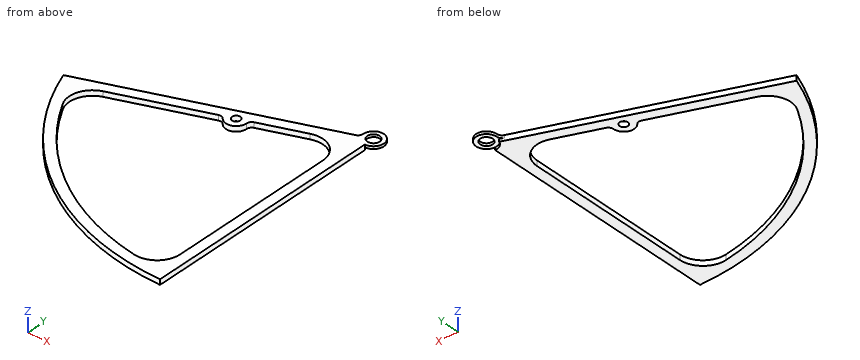
```python
from build123d import *

# Parameters (mm, degrees)
SZKIC1_R                    = 12
SZKIC1_R_2                  = 8
DODANIE_WYCI_GNI_CIE1_DEPTH = 10
SZKIC2_R                    = 20
WYTNIJ_WYCI_GNI_CIE1_DEPTH  = 5
ZAOKR_GLENIE1_R             = 45
ZAOKR_GLENIE2_R             = 10


with BuildPart() as part:
    # Szkic1 → Dodanie-wyciągnięcie1 (new body)
    with BuildSketch(Plane.XY):
        with BuildLine():
            Line((0, -20), (0, -490))
            ThreePointArc((0, -490), (-281.052453812, -401.384501702), (-460.449384185, -167.58987023))
            Line((-460.449384185, -167.58987023), (-18.793852416, -6.840402867))
            ThreePointArc((-18.793852416, -6.840402867), (11.471528727, 16.383040886), (0, -20))
        make_face()
        Circle(SZKIC1_R, mode=Mode.SUBTRACT)
        with Locations((-190.094997116, -90.472476083)):
            Circle(SZKIC1_R_2, mode=Mode.SUBTRACT)
        with BuildLine():
            Line((-20, -28.562960135), (-20, -469.574275275))
            ThreePointArc((-20, -469.574275275), (-269.580925085, -385.001460816), (-434.41507852, -179.397713347))
            Line((-434.41507852, -179.397713347), (-208.888849532, -97.312878949))
            ThreePointArc((-208.888849532, -97.312878949), (-183.254594249, -109.266328498), (-171.3011447, -83.632073216))
            Line((-171.3011447, -83.632073216), (-20, -28.562960135))
        make_face(mode=Mode.SUBTRACT)
    extrude(amount=DODANIE_WYCI_GNI_CIE1_DEPTH)

    # Szkic2 → Wytnij-wyciągnięcie1 (cut)
    with BuildSketch(Plane(origin=(0, 0, 0), x_dir=(-1, 0, 0), z_dir=(0, 0, -1))):
        Circle(SZKIC2_R)
    extrude(amount=-WYTNIJ_WYCI_GNI_CIE1_DEPTH, mode=Mode.SUBTRACT)

    # Zaokrąglenie1
    zaokr_glenie1_edges = [part.edges().sort_by_distance(p)[0] for p in [
        (-434.41507852, -179.397713347, 5),
        (-20, -469.574275275, 5),
        (-20, -28.562960135, 5),
    ]]
    fillet(zaokr_glenie1_edges, radius=ZAOKR_GLENIE1_R)

    # Zaokrąglenie2
    zaokr_glenie2_edges = [part.edges().sort_by_distance(p)[0] for p in [
        (-171.3011447, -83.632073216, 5),
        (-208.888849532, -97.312878949, 5),
        (-18.793852416, -6.840402867, 7.5),
    ]]
    fillet(zaokr_glenie2_edges, radius=ZAOKR_GLENIE2_R)


solid = part.part
```
Model file for the job. Use its own axes, mm. Round coordinates to 2 decimals unless told otherwise and drop trailing zeros. Loops run counter-clockwise (first coordinate to the right, second up) from the corner with the lowest first, then second, coordinate; pieces in that order, holes last. Notation, with made-up numbers: M -18.75,71 L -4.75,71 A33 cw -4.75,109 Z; hole C 66,65 d7. An arc over 180 degrees is marked long. Put each result on its own line as item: value. Start each with the question number.
Item 1: Drop flat-ended pins along their axis: P1, Ø1.5, axis at y = -365.5, z = 9, coming from the +X side; P2, Ø1.5, axis at x = -45, z = 6, coming from the -Y side; P3, Ø1.5, axis at x = -100.5, z = 3, coming from the -Y side. Give the stop position or say it passes through.
Item 2: Cut at A-A (y = -438.5). List the corners of the cut face in (x, z), then the cut area to 3 significant figures.
Item 3: Cut at C-C (y = -208.5). List the corners of the cut face in (x, z), then the cut area to 3 significant figures.
Item 4: Drill centre lines: line 1 along X through (y, z) = (0, 6.65); line 2 along Y through (x, z) = (-144.5, 0.5); line 3 along Y through (x, z) = (-372.5, 7.75). Where is each one in solid material? Low to high.
Item 5: Cut at B-B (z = 7.25). List the corners of the cut face in (x, y) (1 decimal), then the cut area to 3 significant figures.
Answer block:
1. P1: x = 0
1. P2: y = -488
1. P3: y = -479.74
2. outline: M -218.67,0 L -169.17,0 L -169.17,10 L -218.67,10 Z; M -23.98,0 L 0,0 L 0,10 L -23.98,10 Z
2. area: 735 mm2
3. outline: M -443.43,0 L -417.28,0 L -417.28,10 L -443.43,10 Z; M -20,0 L 0,0 L 0,10 L -20,10 Z
3. area: 461 mm2
4. line 1: -20 to -12, 12 to 20
4. line 2: -468.21 to -447.24, -73.88 to -52.59
4. line 3: -318.35 to -286.61, -156.86 to -135.58
5. outline: M -460.4,-167.6 A490 ccw 0,-490 L 0,-20 A20 ccw long -20,-0.2 A10 cw -26.6,-9.7 Z; hole M -411.9,-226.4 A470 ccw -71.9,-464.5 A45 ccw -20,-420 L -20,-92.8 A45 ccw -80.4,-50.5 L -163.5,-80.8 A10 ccw -170.1,-90.3 A20 cw -205.5,-103.2 A10 ccw -216.7,-100.1 L -387.8,-162.4 A45 ccw Z; hole C -190.1,-90.5 d16; hole C 0,0 d24
5. area: 33,100 mm2
